from build123d import *

# Parameters (mm, degrees)
SKETCH3_R          = 1
CUT_EXTRUDE2_DEPTH = 4
SKETCH6_R          = 1
CUT_EXTRUDE3_DEPTH = 3


with BuildPart() as part:
    # Sketch2 → Revolve1 (revolve)
    with BuildSketch(Plane.XY, mode=Mode.PRIVATE) as revolve1_sk:
        Polygon((0, 0), (1, 0), (1, 1.8), (9.5, 1.8), (11.5, 3.8), (11.5, 4.8), (11, 4.8), (11, 5.3), (11.5, 5.3), (11.5, 6.3), (9.5, 6.3), (9.5, 6.6), (11.5, 6.6), (11.5, 16.8), (8, 20.3), (1, 20.3), (1, 23.8), (0, 23.8), align=None)
        Polygon((2, 19.3), (7.585786438, 19.3), (10.5, 16.385786438), (10.5, 12.3), (1, 12.3), (1, 18.3), (2, 18.3), align=None, mode=Mode.SUBTRACT)
    revolve(revolve1_sk.sketch.rotate(Axis((0, 23.8, 0), (0, -1, 0)), 180), axis=Axis((0, 23.8, 0), (0, -1, 0)))

    # Sketch3 → Cut-Extrude2 (cut)
    with BuildSketch(Plane(origin=(0, 20.3, 0), x_dir=(1, 0, 0), z_dir=(0, 1, 0))):
        with Locations(Location((0, 4.5, 0), (0, 0, 180))):
            Circle(SKETCH3_R)
        with Locations(Location((4.5, 0, 0), (0, 0, 180))):
            Circle(SKETCH3_R)
        with Locations(Location((0, -4.5, 0), (0, 0, 180))):
            Circle(SKETCH3_R)
        with Locations(Location((-4.5, 0, 0), (0, 0, 180))):
            Circle(SKETCH3_R)
        with BuildLine():
            Line((-3, 9), (-3, 18.567871813))
            Line((-3, 18.567871813), (3, 18.567871813))
            Line((3, 18.567871813), (3, 9))
            ThreePointArc((3, 9), (0, 6), (-3, 9))
        make_face()
        with BuildLine():
            Line((6.294228634, 7.098076211), (14.580248685, 11.882012118))
            Line((14.580248685, 11.882012118), (17.580248685, 6.685859695))
            Line((17.580248685, 6.685859695), (9.294228634, 1.901923789))
            ThreePointArc((9.294228634, 1.901923789), (5.196152423, 3), (6.294228634, 7.098076211))
        make_face()
        with BuildLine():
            Line((9.294228634, -1.901923789), (17.580248685, -6.685859695))
            Line((17.580248685, -6.685859695), (14.580248685, -11.882012118))
            Line((14.580248685, -11.882012118), (6.294228634, -7.098076211))
            ThreePointArc((6.294228634, -7.098076211), (5.196152423, -3), (9.294228634, -1.901923789))
        make_face()
        with BuildLine():
            Line((3, -9), (3, -18.567871813))
            Line((3, -18.567871813), (-3, -18.567871813))
            Line((-3, -18.567871813), (-3, -9))
            ThreePointArc((-3, -9), (0, -6), (3, -9))
        make_face()
        with BuildLine():
            Line((-6.294228634, -7.098076211), (-14.580248685, -11.882012118))
            Line((-14.580248685, -11.882012118), (-17.580248685, -6.685859695))
            Line((-17.580248685, -6.685859695), (-9.294228634, -1.901923789))
            ThreePointArc((-9.294228634, -1.901923789), (-5.196152423, -3), (-6.294228634, -7.098076211))
        make_face()
        with BuildLine():
            Line((-9.294228634, 1.901923789), (-17.580248685, 6.685859695))
            Line((-17.580248685, 6.685859695), (-14.580248685, 11.882012118))
            Line((-14.580248685, 11.882012118), (-6.294228634, 7.098076211))
            ThreePointArc((-6.294228634, 7.098076211), (-5.196152423, 3), (-9.294228634, 1.901923789))
        make_face()
    extrude(amount=-CUT_EXTRUDE2_DEPTH, mode=Mode.SUBTRACT)

    # Sketch6 → Cut-Extrude3 (cut)
    with BuildSketch(Plane.XZ.offset(-1.8)):
        with Locations((0, 6)):
            Circle(SKETCH6_R)
        with Locations((8, 0)):
            Circle(SKETCH6_R)
        with Locations((0, -6)):
            Circle(SKETCH6_R)
        with Locations((-8, 0)):
            Circle(SKETCH6_R)
    extrude(amount=-CUT_EXTRUDE3_DEPTH, mode=Mode.SUBTRACT)


solid = part.part
Read the model definition and answer for the solid it produces. Units are mm, in the model's axes. A direction names the side the tool comes from. Round coordinates to 2 decimals unless told otherwise and drop trailing zeros. Order: outer loops, then holes, each group sorted by start corner. A loop starts at its lowest first (then second) coordinate and runs counter-clockwise, first axis right, second up.
1) Straight lines are drawn through the part: L1, parallel to Y at x = -1.75, z = -4.25; L2, parallel to Y at x = 10.25, z = -4.75; L3, parallel to Y at x = -6.5, z = 9.25. For each, find the intervals that lie inside material, in ascending order.
2) The part is cut by section B-B on y = 19.75. Write down the section's boundary in (x, z).
3) Flat-ended cylindrical pins translate along their axes: pin 1 (0.7 mm diameter, centred on x = 0, z = 10.5, fed in from +Y); pin 2 (2.5 mm diameter, centred on x = 0, z = 4.5, fed in from -Y); pin 3 (8 mm diameter, centred on x = -9, y = 10, fed in from -Z). Find the tip coordinate at first contact, or state that the pin passes through.
4) The part is cut by section A-A on y = 14.5. Write down the section's boundary in (x, z).
5) The part is cut by section C-C on z = -4.5. Give the number of separate pieces and of enclosed holes in the cut face, plus the area to 3 significant figures.
6) For faces 1 (the face through (5.23, 19.51, -2.94)), 2 (the face through (10.015, 17.295, -2.318)), 3 (the face through (-6.99, 17.29, 7.5)), 4 (the face through (0, 3, -5)), determine the directions among +Z, -Z, +X, -X, +Y, -Y from which every point of the face is accessible in a straight line to the end or side of a thin tool.
7) The mould has two halves that part along Z. Classify faces 5 (the face through (0, 1, 1)), 6 (the face through (4.832, 18.574, -8.44)), 7 (the face through (0, 4.8, 6)): released by +Z, released by -Z, zero draft, split by the parting line, or undercut.
Resolved:
1. L1: y = 1.8 to 12.3, 19.3 to 20.3
1. L2: y = 3.6 to 4.8, 5.3 to 6.3, 6.6 to 16.3
1. L3: y = 3.61 to 4.8, 5.3 to 6.3, 6.6 to 16.99
2. outline: (-8.41, -1.56) arc R3 cw to (-5.56, -6.5) arc R8.55 ccw to (-2.85, -8.06) arc R3 cw to (2.85, -8.06) arc R8.55 ccw to (5.56, -6.5) arc R3 cw to (8.41, -1.56) arc R8.55 ccw to (8.41, 1.56) arc R3 cw to (5.56, 6.5) arc R8.55 ccw to (2.85, 8.06) arc R3 cw to (-2.85, 8.06) arc R8.55 ccw to (-5.56, 6.5) arc R3 cw to (-8.41, 1.56) arc R8.55 ccw to start; hole circle Ø2 at (-4.5, 0); hole circle Ø2 at (0, -4.5); hole circle Ø2 at (0, 4.5); hole circle Ø2 at (4.5, 0)
3. pin 1: stops at y = 16.3
3. pin 2: stops at y = 1.8
3. pin 3: stops at z = -10.36
4. outline: circle Ø23 at (0, 0); circle Ø2 at (0, 0); hole circle Ø21 at (0, 0)
5. separate pieces: 3
5. enclosed holes: 0
5. area: 232 mm2
6. face 1: +Y
6. face 2: -Z, +Y
6. face 3: -X, +Y
6. face 4: -Y
7. face 5: split by the parting line
7. face 6: released by -Z
7. face 7: undercut
